The listing builds one solid part. Answer for the finished solid, in the listing's coordinates (mm). Face numbers are marked on the shaded views. A direction names the side the tool comes from. Coordinates: 2 decimals unless noted, no trailing zeros. Write each loop counter-clockwise with the first axis right and the second up, starting at its lowest first coordinate (ties: lowest second). Pieces come first, ordered by that corner, then holes. Notation, with made-up numbers: M 73.5,71.25 L 101.5,71.25 A28 cw 101.5,110.25 Z; hole C 45,79 d7. An arc over 180 degrees is marked long. Answer as CSV lines item,"result".
Autodesk Inventor part; units mm, degrees
ref_plane "insert_XY" through (0, 0, 0) normal (0, 1, 0) x (1, 0, 0)
ref_plane "insert_YZ" through (0, 0, 0) normal (1, 0, 0) x (0, 0, -1)
ref_plane "insert_ZX" through (0, 0, 0) normal (0, 0, -1) x (0, 1, 0)
sketch "Sketch_1" plane through (0, 0, 0) normal (0, 0, 1) x (1, 0, 0)
  line L0 (0, -1.27) -> (0, 6.858)
  line L1 (0, 6.858) -> (3.0861, 6.858)
  line L2 (3.0861, 6.858) -> (3.0861, 0)
  line L3 (3.0861, 0) -> (6.35, 0)
  line L4 (6.35, 0) -> (6.35, -1.27)
  line L5 (6.35, -1.27) -> (0, -1.27)
  line L6 (0, -1.27) -> (0, 6.858)
revolve "Revolution1" add sketch "Sketch_1" angle 360 about axis through (0, -1.27, 0) along (0, -1, 0)
sketch "Sketch2" plane through (0, -1.27, 0) normal (0, -1, 0) x (1, 0, 0)
  point P0 (0, 0)
hole "Drilling 1" at (0, -1.27, 0) direction (0, 1, 0) diameter 3.9624 depth 8.128 countersink diameter 4.826 countersink angle 90
sketch "Sketch_3" plane through (0, 0, 0) normal (0, 1, 0) x (-1, 0, 0)
  circle A0 centre (0, 0) radius 8.89
  line L0 (6.35, 0) -> (4.826, 0)
  line L1 (4.826, 0) -> (4.826, 4.127)
  arc A1 (4.826, 4.127) -> (-3.175, 5.4993) centre (0, 0) ccw
  line L2 (-3.175, 5.4993) -> (-2.413, 4.1794)
  line L3 (-2.413, 4.1794) -> (-5.9871, 2.1159)
  arc A2 (-5.9871, 2.1159) -> (-3.175, -5.4993) centre (0, 0) ccw
  line L4 (-3.175, -5.4993) -> (-2.413, -4.1794)
  line L5 (-2.413, -4.1794) -> (1.1611, -6.2429)
  arc A3 (1.1611, -6.2429) -> (6.35, 0) centre (0, 0) ccw
extrude "Extrusion1" cut sketch "Sketch_3" against normal blind 2.54
ref_plane "insert_XY" through (0, 0, 0) normal (0, 1, 0) x (1, 0, 0)
ref_plane "insert_YZ" through (0, 0, 0) normal (1, 0, 0) x (0, 0, -1)
ref_plane "insert_ZX" through (0, 0, 0) normal (0, 0, -1) x (0, 1, 0)
properties part number "6895_insert" material "Stainless Steel"
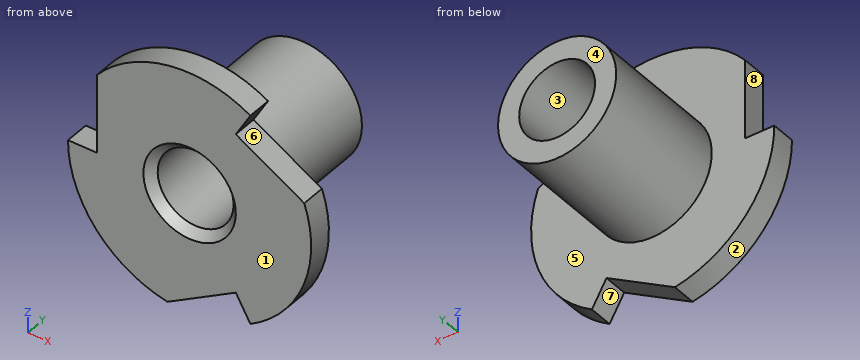
Q1. For the marked faces 4, 5, 6, 7 and 8, determine the directions among +Z, -Z, +X, -X, +Y, -Y from which every point of the face is accessible in a straight line to the end or side of a thin tool.
Output:
face 4,"+Z, -Z, +X, -X, +Y"
face 5,"+Y"
face 6,"+X, +Y, -Y"
face 7,"-Z, +Y, -Y"
face 8,"+Z, -X, +Y, -Y"
Q2. Straight lines are drawn through the part: line 1 (Z direction, x = 0, y = 2.5); line 2 (Y direction, x = -4.5, z = -0.5); line 3 (X direction, y = 3.75, z = 0.75). For each, find the intervals that lie inside material, in ascending order.
Output:
line 1,"-3.09 to -1.98, 1.98 to 3.09"
line 2,"-1.27 to 0"
line 3,"-2.99 to -1.83, 1.83 to 2.99"
Q3. Find section D-D (x = 5.75). Give the vertices of the cut face in (y, z).
Output:
outline,"M -1.27,-2.69 L 0,-2.69 L 0,2.25 L -1.27,2.25 Z"
Q4. Flat-ended cylindrical pins translate along their axes: pin 1 Ø0.6 at (y, z) = (-1, 1) entering from -X; pin 2 Ø1 at (x, z) = (1, -3.5) entering from +Y; pin 3 Ø3 at (x, y) = (-3.5, 5.5) entering from -Z; pin 4 Ø2.5 at (x, z) = (0, 0) entering from -Y. Find the tip coordinate at first contact, or state that the pin passes through.
Output:
pin 1,"x = -4.83"
pin 2,"y = 0"
pin 3,"z = -2.35"
pin 4,"through"
Q5. Find section A-A (x = 0). Give the vertices of the cut face in (y, z).
Output:
outline,"M -1.27,-5.57 L 0,-5.57 L 0,-3.09 L 6.86,-3.09 L 6.86,-1.98 L -0.84,-1.98 L -1.27,-2.41 Z; M -1.27,2.41 L -0.84,1.98 L 6.86,1.98 L 6.86,3.09 L 0,3.09 L 0,6.35 L -1.27,6.35 Z"
Q6. The mould has two halves that part along X. Classify the marked faces 1, 2 and 3: pulls with the +X half, pulls with the -X half, needs draft (parallel to the pull), parting line crosses it, or undercut.
Output:
face 1,"needs draft"
face 2,"pulls with the -X half"
face 3,"undercut"
Q7. Find section C-C (y = 3.75). Give the vertices of the cut face in (x, z).
Output:
outline,"C 0,0 d6.17; hole C 0,0 d3.96"
Q8. Find section B-B (z = -5.25). Give the vertices of the cut face in (x, y), and give its area (3 significant figures).
Output:
outline,"M -3.57,-1.27 L 0.56,-1.27 L 0.56,0 L -3.57,0 Z; M 3.03,-1.27 L 3.57,-1.27 L 3.57,0 L 3.03,0 Z"
area,"5.93 mm2"
